The model under review builds one solid part; all positions refer to its coordinate system, in mm. A direction names the side the tool comes from. Coordinates: 2 decimals unless noted, no trailing zeros. Write each loop counter-clockwise with the first axis right and the second up, starting at its lowest first coordinate (ties: lowest second). Pieces come first, ordered by that corner, then holes. Notation, with made-up numbers: (7, 17) - (48, 17) arc R22 ccw to (48, 34) - close; hole circle Ø3 at (-37.5, -31.5). An arc over 180 degrees is marked (long way). Put each result on its own line as item: value.
from build123d import *
from build123d.topology import SkipClean

# Parameters (mm, degrees)
SKETCH_1_R      = 1.1
SKETCH_1_W      = 47
SKETCH_1_H      = 44
EXTRUDE_1_DEPTH = 1
EXTRUDE_START   = 2.25
SKETCH_2_R      = 1.1
SKETCH_2_W      = 51.5
SKETCH_2_H      = 46.5
EXTRUDE_2_DEPTH = 2.25
CHAMFER_1_SIZE  = 1.6
CHAMFER_1_SIZE2 = 0.923760431
FILLET_1_R      = 1


with BuildPart() as part:
    # 草图1 → 凸台-拉伸1 (new body)
    with BuildSketch(Plane.XY):
        with BuildLine():
            Line((-26.5, -26.5), (26.5, -26.5))
            ThreePointArc((26.5, -26.5), (28.267766953, -25.767766953), (29, -24))
            Line((29, -24), (29, 24))
            ThreePointArc((29, 24), (28.267766953, 25.767766953), (26.5, 26.5))
            Line((26.5, 26.5), (-26.5, 26.5))
            ThreePointArc((-26.5, 26.5), (-28.267766953, 25.767766953), (-29, 24))
            Line((-29, 24), (-29, -24))
            ThreePointArc((-29, -24), (-28.267766953, -25.767766953), (-26.5, -26.5))
        make_face()
        with Locations((-26.9, 24.4)):
            Circle(SKETCH_1_R, mode=Mode.SUBTRACT)
        with Locations(Location((26.9, 24.4, 0), (0, 0, 180))):
            Circle(SKETCH_1_R, mode=Mode.SUBTRACT)
        with Locations(Location((-26.9, -24.4, 0), (0, 0, 180))):
            Circle(SKETCH_1_R, mode=Mode.SUBTRACT)
        with Locations((26.9, -24.4)):
            Circle(SKETCH_1_R, mode=Mode.SUBTRACT)
        Rectangle(SKETCH_1_W, SKETCH_1_H, mode=Mode.SUBTRACT)
    extrude(amount=EXTRUDE_1_DEPTH)

    # 草图2 → 凸台-拉伸2 (add)
    with SkipClean():  # the faces are left unmerged after this step: merging them gives an invalid solid
        with BuildSketch(Plane(origin=(0, 0, 0), x_dir=(-1, 0, 0), z_dir=(0, 0, -1)).offset(EXTRUDE_START)):
            with BuildLine():
                Line((26.5, 26.5), (-26.5, 26.5))
                ThreePointArc((-26.5, 26.5), (-28.267766953, 25.767766953), (-29, 24))
                Line((-29, 24), (-29, -24))
                ThreePointArc((-29, -24), (-28.267766953, -25.767766953), (-26.5, -26.5))
                Line((-26.5, -26.5), (26.5, -26.5))
                ThreePointArc((26.5, -26.5), (28.267766953, -25.767766953), (29, -24))
                Line((29, -24), (29, 24))
                ThreePointArc((29, 24), (28.267766953, 25.767766953), (26.5, 26.5))
            make_face()
            with Locations((26.9, -24.4)):
                Circle(SKETCH_2_R, mode=Mode.SUBTRACT)
            with Locations((-26.9, -24.4)):
                Circle(SKETCH_2_R, mode=Mode.SUBTRACT)
            with Locations((-26.9, 24.4)):
                Circle(SKETCH_2_R, mode=Mode.SUBTRACT)
            with Locations((26.9, 24.4)):
                Circle(SKETCH_2_R, mode=Mode.SUBTRACT)
            Rectangle(SKETCH_2_W, SKETCH_2_H, mode=Mode.SUBTRACT)
        extrude(amount=-EXTRUDE_2_DEPTH)

    # 倒角1
    chamfer_1_edges = [part.edges().sort_by_distance(p)[0] for p in [
        (-23.5, 0, 1),
        (0, -22, 1),
        (23.5, 0, 1),
        (0, 22, 1),
    ]]
    chamfer_1_side = [part.faces().sort_by_distance(p)[0] for p in [
        (0, -25.714315585, 1),
    ]]
    chamfer(chamfer_1_edges, length=CHAMFER_1_SIZE, length2=CHAMFER_1_SIZE2, reference=chamfer_1_side[0])

    # 圆角1
    fillet_1_edges = [part.edges().sort_by_distance(p)[0] for p in [
        (0, 23.6, 1),
        (25.1, 0, 1),
        (0, -23.6, 1),
        (-25.1, 0, 1),
        (24.3, 22.8, 0.538119785),
        (24.3, -22.8, 0.538119785),
        (-24.3, 22.8, 0.538119785),
        (-24.3, -22.8, 0.538119785),
    ]]
    fillet(fillet_1_edges, radius=FILLET_1_R)


solid = part.part
1. Consider section B-B on x = -9.5. State the section outline as (y, z) points, plus the area to 3 significant figures.
Determined:
outline: (-26.5, -2.25) - (-23.25, -2.25) - (-23.25, 0) - (-22, 0) - (-22, 0.08) - (-23.37, 0.87) arc R1 ccw to (-23.87, 1) - (-26.5, 1) - close; (22, 0) - (23.25, 0) - (23.25, -2.25) - (26.5, -2.25) - (26.5, 1) - (23.87, 1) arc R1 ccw to (23.37, 0.87) - (22, 0.08) - close
area: 22.1 mm^2
2. For pin 1 Ø1.8 at (x, y) = (-26.9, -24.4) entering from +Z, flat-tipped, find the tip position at first contact; note if it passes through.
Determined:
pin 1: passes through
3. Consider section A-A on y = 0. State the section outline as (x, z) points.
Determined:
outline: (-29, -2.25) - (-25.75, -2.25) - (-25.75, 0) - (-23.5, 0) - (-23.5, 0.08) - (-24.87, 0.87) arc R1 ccw to (-25.37, 1) - (-29, 1) - close; (23.5, 0) - (25.75, 0) - (25.75, -2.25) - (29, -2.25) - (29, 1) - (25.37, 1) arc R1 ccw to (24.87, 0.87) - (23.5, 0.08) - close
4. To check wall thickness, follow probe 1 along X at (y, z) = (24.4, -1.55); probe 2 along X at (y, z) = (24.5, 0.75); probe 3 along Y at (x, z) = (-26.9, 0.7). State the ranges of each line that lie inside material, in increasing order.
Determined:
probe 1: x = -28.97 to -28, -25.8 to 25.8, 28 to 28.97
probe 2: x = -28.95 to -28, -25.8 to 25.8, 28 to 28.95
probe 3: y = -26.47 to -25.5, -23.3 to 23.3, 25.5 to 26.47
5. The part is to be moulded in two halves that separate along X. For faces 1 (the cylindrical face through (-24.04, 22.547, 0.465)), 2 (the flat face through (29, 0, -1)), 3 (the flat face through (0, 26, 1)), say which applies: +X half, -X half, draft (parallel to the pull), parting line (faces both ways), or undercut.
Determined:
face 1: undercut
face 2: +X half
face 3: draft
6. Machinability: for faces 4 (the flat face through (-2, -22.3, 0)), 5 (the cylindrical face through (28, -26, -1)), 6 (the cylindrical face through (24.047, -22.54, 0.465)), which of the approach directions +Z, -Z, +X, -X, +Y, -Y give a long, thin tool a straight path to every point of the face, cutting with its end or side? Answer none if there is none.
Determined:
face 4: -Z
face 5: +Z, -Z, +X, -Y
face 6: +Z
7. Consider section C-C on z = -0.6. State the section outline as (x, y) points.
Determined:
outline: (-29, -24) arc R2.5 ccw to (-26.5, -26.5) - (26.5, -26.5) arc R2.5 ccw to (29, -24) - (29, 24) arc R2.5 ccw to (26.5, 26.5) - (-26.5, 26.5) arc R2.5 ccw to (-29, 24) - close; hole circle Ø2.2 at (-26.9, -24.4); hole circle Ø2.2 at (-26.9, 24.4); hole (-25.75, -23.25) - (25.75, -23.25) - (25.75, 23.25) - (-25.75, 23.25) - close; hole circle Ø2.2 at (26.9, -24.4); hole circle Ø2.2 at (26.9, 24.4)
